The model under review builds one solid part; all positions refer to its coordinate system, in mm. A direction names the side the tool comes from. Round coordinates to 2 decimals unless told otherwise and drop trailing zeros. Return JSON: item names as keys, results as strings. Group by question number.
1. Mouldability with a two-part tool opening along Z and no side actions: class faces 6 (the flat face through (-2.5, -2.5, -11.405)), 7 (the flat face through (8.8, 5.796, -5.134)), 8 (the cylindrical face through (0.69, -3.1, -5.42)) as pulls with the +Z half, pulls with the -Z half, needs draft (parallel to the pull), parting line crosses it, or undercut.
2. For line 1 along Y through (x, z) = (0, -8.5) (3 decimals); line 2 along Z through (x, y) = (-9.75, -3); line 3 along Z through (x, y) = (-10.5, 1), list the stretches that pass through material, from the lowest coordinate up. Write a range as from..to.
3. Tool access review of faces 1 (the flat face through (7.542, 7.398, -5.134)), 2 (the flat face through (-1.08, 10.51, -5.13)), 3 (the cylindrical face through (6.889, -8.655, -5.134)), 4 (the flat face through (8, -7, -10.414)), 5 (the flat face through (-10.02, 3.27, -5.13)): name each direction out of +Z, -Z, +X, -X, +Y, -Y from which nothing blocks a thin tool from reaching the whole face with its end or side.
4. Clearance check with flat-ended pins moving along their axes: P1, Ø0.5, axis at x = 10, y = 2.5, coming from the +Z side; P2, Ø5, axis at y = -4.5, z = -1.5, coming from the -X side; P3, Ø1.7, axis at x = -10.5, y = 3, coming from the +Z side. State where each tip first meets the part, or that it passes through.
from build123d import *

# Parameters (mm, degrees)
SKETCH1_R           = 11.0617
BASEPULLEY_DEPTH    = 10.414
GROOVE_DEPTH        = 5.207
GROOVES_COUNT       = 14
GROOVES_ANGLE       = 334.285714286
SKETCH4_W           = 0.254
SKETCH4_H           = 11.43
BORSKE_R            = 3.175
BORE_DEPTH          = 21.970083094
BOSS_EXTRUDE1_START = 0.254
SKETCH7_R           = 11.992065176
SKETCH7_R_2         = 3.175
BOSS_EXTRUDE1_DEPTH = 0.254


with BuildPart() as part:
    # Sketch1 → BasePulley (new body)
    with BuildSketch(Plane.XY):
        Circle(SKETCH1_R)
    extrude(amount=-BASEPULLEY_DEPTH)

    # Sketch2 → Flange (revolve)
    with BuildSketch(Plane(origin=(0, 0, 0), x_dir=(0, 0, -1), z_dir=(1, 0, 0)), mode=Mode.PRIVATE) as flange_sk:
        Polygon((10.414, 11.0617), (10.724622372, 12.0777), (11.429036456, 11.862339002), (11.1506, 10.951614392), (11.1506, 0), (-0.7366, 0), (-0.7366, 10.951614392), (-1.015036456, 11.862339002), (-0.310622372, 12.0777), (0, 11.0617), align=None)
    revolve(flange_sk.sketch.rotate(Axis((0, 0, 0), (0, 0, -1)), 90), axis=Axis((0, 0, 0), (0, 0, -1)))

    # Sketch3 → Groove (cut, symmetric)
    with BuildSketch(Plane.XY.offset(-5.207)):
        with BuildLine():
            Line((-1.2827, 11.0617), (-1.2827, 36.4617))
            Line((-1.2827, 36.4617), (1.2827, 36.4617))
            Line((1.2827, 36.4617), (1.2827, 11.0617))
            Line((1.2827, 11.0617), (0.659450384, 9.9822))
            ThreePointArc((0.659450384, 9.9822), (0.519994706, 9.842744321), (0.329494706, 9.7917))
            Line((0.329494706, 9.7917), (-0.55367873, 9.7917))
            ThreePointArc((-0.55367873, 9.7917), (-0.772211353, 9.860603071), (-0.911701619, 10.042390325))
            Line((-0.911701619, 10.042390325), (-1.2827, 11.0617))
        make_face()
    groove = extrude(amount=GROOVE_DEPTH, both=True, mode=Mode.SUBTRACT)

    # Grooves: Groove ×14 about axis
    grooves_axis = Axis((0, 0, -10.414), (0, 0, 1))
    for i in range(1, GROOVES_COUNT):
        add(groove.rotate(grooves_axis, i * GROOVES_ANGLE / (GROOVES_COUNT - 1)), mode=Mode.SUBTRACT)

    # Sketch4 → BaseHub (revolve)
    with BuildSketch(Plane(origin=(0, 0, 0), x_dir=(0, 0, -1), z_dir=(1, 0, 0)), mode=Mode.PRIVATE) as basehub_sk:
        with Locations((-0.127, 5.715)):
            Rectangle(SKETCH4_W, SKETCH4_H)
    revolve(basehub_sk.sketch.rotate(Axis((0, 0, 0), (0, 0, -1)), 90), axis=Axis((0, 0, 0), (0, 0, -1)))

    # BorSke → Bore (cut, through all)
    with BuildSketch(Plane(origin=(0, 0, -11.1506), x_dir=(-1, 0, 0), z_dir=(0, 0, -1))):
        Circle(BORSKE_R)
    extrude(amount=-BORE_DEPTH, mode=Mode.SUBTRACT)

    # Sketch7 → Boss-Extrude1 (add)
    with BuildSketch(Plane(origin=(0, 0, -11.1506), x_dir=(-1, 0, 0), z_dir=(0, 0, -1)).offset(BOSS_EXTRUDE1_START)):
        Circle(SKETCH7_R)
        Circle(SKETCH7_R_2, mode=Mode.SUBTRACT)
    extrude(amount=-BOSS_EXTRUDE1_DEPTH)


solid = part.part
Output:
{
 "1": {"face 6": "pulls with the -Z half", "face 7": "undercut", "face 8": "needs draft"},
 "2": {"line 1": "y = -9.792..-3.175, 3.175..9.792", "line 2": "z = -11.4..-10.41, 0..0.74", "line 3": "z = -11.4..0.74"},
 "3": {"face 1": "+X", "face 2": "+Y", "face 3": "+X, -Y", "face 4": "none", "face 5": "-X"},
 "4": {"P1": "stops at z = 0.74", "P2": "stops at x = -11.75", "P3": "stops at z = 0.99"}
}
